from build123d import *

# Parameters (mm, degrees)
SKETCH1_R           = 2.54
BOSS_EXTRUDE1_DEPTH = 1.016


with BuildPart() as part:
    # Sketch1 → Boss-Extrude1 (new, symmetric)
    with BuildSketch(Plane.XY):
        Polygon((76.2, 3.175), (76.2, 22.225), (73.025, 25.4), (44.45, 25.4), (25.4, 44.45), (25.4, 73.025), (22.225, 76.2), (3.175, 76.2), (0, 73.025), (0, 3.175), (3.175, 0), (73.025, 0), align=None)
        with Locations((12.7, 12.7)):
            Circle(SKETCH1_R, mode=Mode.SUBTRACT)
        with Locations((12.7, 38.1)):
            Circle(SKETCH1_R, mode=Mode.SUBTRACT)
        with Locations((12.7, 63.5)):
            Circle(SKETCH1_R, mode=Mode.SUBTRACT)
        with Locations((38.1, 12.7)):
            Circle(SKETCH1_R, mode=Mode.SUBTRACT)
        with Locations((63.5, 12.7)):
            Circle(SKETCH1_R, mode=Mode.SUBTRACT)
    extrude(amount=BOSS_EXTRUDE1_DEPTH, both=True)


solid = part.part
Read the model definition and answer for the solid it produces. Units are mm, in the model's axes. A direction names the side the tool comes from. Give positions to 0.01 mm unless a question says otherwise; leave off trailing zeros. Loops run counter-clockwise (first coordinate to the right, second up) from the corner with the lowest first, then second, coordinate; pieces in that order, holes last. Notation, with made-up numbers: M 7,44 L 29,44 A28 cw 29,74 Z; hole C -35,62 d8. An arc over 180 degrees is marked long. Write each question's results on one line, items separated by ' | '.
1. Section C-C on z = 0.6 is taken. Give the vertices of the cut face in (x, y) (3 decimals).
Values:
outline: M 0,3.175 L 3.175,0 L 73.025,0 L 76.2,3.175 L 76.2,22.225 L 73.025,25.4 L 44.45,25.4 L 25.4,44.45 L 25.4,73.025 L 22.225,76.2 L 3.175,76.2 L 0,73.025 Z; hole C 12.7,12.7 d5.08; hole C 12.7,38.1 d5.08; hole C 12.7,63.5 d5.08; hole C 38.1,12.7 d5.08; hole C 63.5,12.7 d5.08
2. Given pin 1 (6 mm diameter, centred on x = 12.7, y = 12.7, fed in from +Z); pin 2 (1 mm diameter, centred on x = 64.5, z = -0.5, fed in from +Y), each flat-ended and moving along its own axis, determine where each tip first touches the part or whether it passes through.
Values:
pin 1: stops at z = 1.02 | pin 2: stops at y = 25.4
3. The mould has two halves that part along X. Classify faces 1 (the face through (38, 0, 0)), 2 (the face through (65.923, 13.463, -0.014)), 3 (the face through (74.59, 1.565, 0.014)): pulls with the +X half, pulls with the -X half, needs draft (parallel to the pull), parting line crosses it, or undercut.
Values:
face 1: needs draft | face 2: undercut | face 3: pulls with the +X half
4. Section A-A on x = 63.5 is taken. Give the vertices of the cut face in (y, z).
Values:
outline: M 0,-1.02 L 10.16,-1.02 L 10.16,1.02 L 0,1.02 Z; M 15.24,-1.02 L 25.4,-1.02 L 25.4,1.02 L 15.24,1.02 Z
5. Straight lines are drawn through the part: line 1 (Y direction, x = 12.7, z = -0.3); line 2 (Y direction, x = 53.5, z = 0.6). For each, find the intervals that lie inside material, in ascending order. Write a range as [from, to].
Values:
line 1: y = [0, 10.16], [15.24, 35.56], [40.64, 60.96], [66.04, 76.2] | line 2: y = [0, 25.4]
6. Section B-B on y = 38.1 is taken. Give the vertices of the cut face in (x, z), plus the area to 3 significant figures.
Values:
outline: M 0,-1.02 L 10.16,-1.02 L 10.16,1.02 L 0,1.02 Z; M 15.24,-1.02 L 31.75,-1.02 L 31.75,1.02 L 15.24,1.02 Z | area: 54.2 mm^2
7. A tool of negligible diameter and unlimited length cuts with its end or side. For faces 4 (the face through (13, 76.2, 0)), 5 (the face through (25.4, 59, 0)), from which of +Z, -Z, +X, -X, +Y, -Y can it reach the whole face along a straight path? Write none if from no direction.
Values:
face 4: +Z, -Z, +X, -X, +Y | face 5: +Z, -Z, +X, +Y
8. Section D-D on y = 12.7 is taken. Give the vertices of the cut face in (x, z).
Values:
outline: M 0,-1.02 L 10.16,-1.02 L 10.16,1.02 L 0,1.02 Z; M 15.24,-1.02 L 35.56,-1.02 L 35.56,1.02 L 15.24,1.02 Z; M 40.64,-1.02 L 60.96,-1.02 L 60.96,1.02 L 40.64,1.02 Z; M 66.04,-1.02 L 76.2,-1.02 L 76.2,1.02 L 66.04,1.02 Z
